from build123d import *

# Parameters (mm, degrees)
F0_R         = 6.35
F1_DEPTH     = 7.62
F2_W         = 7.62
F2_H         = 6.35
F3_DEPTH     = 25.4
F5_DEPTH     = 25.4
F7_DEPTH     = 63.5
F9_DEPTH     = 20.32
F11_DEPTH    = 25.4
F12_R        = 5.08
F13_R        = 0.508
F14_T1_DEPTH = 46.4482991577
F16_DEPTH    = 5.08
F18_DEPTH    = 1.27
F19_T4_DEPTH = 19.0509661188
F20_R        = 0.254


# Not quite as in the source:
# - a fillet or chamfer that OpenCascade refuses, or shapes differently, is made with other operations: its cross-section is extruded or revolved along the edge and cut away or added


with BuildPart() as f1:
    # F0 (on Front) → F1 (new body)
    with BuildSketch(Plane.XZ):
        with BuildLine():
            Line((15.24, 3.81), (9.4185720786, 3.81))
            ThreePointArc((9.4185720786, 3.81), (-10.16, 0), (9.4185720786, -3.81))
            Line((9.4185720786, -3.81), (15.24, -3.81))
            Line((15.24, -3.81), (15.24, 0))
            Line((15.24, 0), (15.24, 3.81))
        make_face()
        Circle(F0_R, mode=Mode.SUBTRACT)
    extrude(amount=F1_DEPTH)

    # F2 (on face) → F3 (join)
    with BuildSketch(Plane.YZ.offset(15.24)):
        Polygon((-7.62, 10.16), (-7.62, 3.81), (-15.24, 3.81), (-15.24, -10.16), (15.24, -10.16), (15.24, 3.81), (15.24, 10.16), align=None)
        with Locations((-11.43, 6.985)):
            Rectangle(F2_W, F2_H)
    extrude(amount=F3_DEPTH)

    # F4 (on face) → F5 (cut)
    with BuildSketch(Plane.XY.offset(10.16)):
        Polygon((31.65983, 15.24), (40.64, 15.24), (40.64, 6.25983), (47.585287597, 13.2393133827), (38.6222154898, 22.2023854898), align=None)
        Polygon((40.64, 6.25983), (40.64, 15.24), (31.65983, 15.24), align=None)
        with BuildLine():
            Line((40.64, 6.25983), (31.65983, 15.24))
            Line((31.65983, 15.24), (22.6795738789, 6.2597438789))
            ThreePointArc((22.6795738789, 6.2597438789), (22.6795738789, -2.7204261211), (31.6597438789, -2.7204261211))
            Line((31.6597438789, -2.7204261211), (40.64, 6.25983))
        make_face()
    extrude(amount=-F5_DEPTH, mode=Mode.SUBTRACT)

    # F6 (on face) → F7 (cut, symmetric)
    with BuildSketch(Plane(origin=(8.209915, -8.209915, 0), x_dir=(0.7071067812, 0.7071067812, 0), z_dir=(0.7071067812, -0.7071067812, 0))):
        with BuildLine():
            ThreePointArc((26.8131878295, 0.635), (24.5681237992, -4.7850640303), (29.9881878295, -2.54))
            ThreePointArc((29.9881878295, -2.54), (29.0582518598, -0.2949359697), (26.8131878295, 0.635))
        make_face()
    extrude(amount=F7_DEPTH, both=True, mode=Mode.SUBTRACT)

    # F8 (on face) → F9 (join)
    with BuildSketch(Plane.XY.offset(10.16)):
        with BuildLine():
            Line((31.6597438789, -2.7204261211), (40.64, 6.25983))
            Line((40.64, 6.25983), (38.8439487758, 8.0558812242))
            Line((38.8439487758, 8.0558812242), (26.2716117366, -4.516455815))
            ThreePointArc((26.2716117366, -4.516455815), (29.177671493, -4.2544271062), (31.6597438789, -2.7204261211))
        make_face()
    extrude(amount=-F9_DEPTH)

    # F10 (on face) → F11 (cut)
    with BuildSketch(Plane(origin=(8.209915, -8.209915, 0), x_dir=(0.7071067812, 0.7071067812, 0), z_dir=(0.7071067812, -0.7071067812, 0))):
        with BuildLine():
            ThreePointArc((29.9881878295, -2.54), (29.0582518598, -0.2949359697), (26.8131878295, 0.635))
            ThreePointArc((26.8131878295, 0.635), (24.5681237992, -4.7850640303), (29.9881878295, -2.54))
        make_face()
    extrude(amount=F11_DEPTH, mode=Mode.SUBTRACT)

    # F12
    f12_edges = [f1.edges().sort_by_distance(p)[0] for p in [
        (40.64, -15.24, 0),
    ]]
    fillet(f12_edges, radius=F12_R)

    # F13
    f13_edges = [f1.edges().sort_by_distance(p)[0] for p in [
        (15.24, -3.81, 3.81),
        (15.24, -3.81, -3.81),
    ]]
    fillet(f13_edges, radius=F13_R)

    # F14: chamfer of 5.08 on 1 edges, made by hand

    # F14_s2 → F14_t1 (cut)
    with BuildSketch(Plane.XY.offset(-23.2241495789)):
        Polygon((15.24, 10.16), (20.32, 15.24), (15.24, 15.24), align=None)
    extrude(amount=F14_T1_DEPTH, mode=Mode.SUBTRACT)

    # F15 (on face) → F16 (join)
    with BuildSketch(Plane.XY.offset(10.16)):
        with BuildLine():
            Line((31.65983, 15.24), (28.3609535545, 15.24))
            Line((28.3609535545, 15.24), (21.4524150836, 8.3314615291))
            ThreePointArc((21.4524150836, 8.3314615291), (19.5659150525, -1.0873397162), (27.5316145271, -6.4557967708))
            Line((27.5316145271, -6.4557967708), (26.2716117366, -4.516455815))
            ThreePointArc((26.2716117366, -4.516455815), (21.1455728938, -0.2383537351), (22.6795738789, 6.2597438789))
            Line((22.6795738789, 6.2597438789), (31.65983, 15.24))
        make_face()
    extrude(amount=F16_DEPTH)

    # F17 (on face) → F18 (cut)
    with BuildSketch(Plane.XY.offset(10.16)):
        Polygon((21.4524150836, 8.3314615291), (28.3609535545, 15.24), (25.7178656757, 15.24), (19.4216053933, 9.3011604622), align=None)
    extrude(amount=-F18_DEPTH, mode=Mode.SUBTRACT)

    # F19: fillet of radius 5.08 on 1 edges, made by hand


with BuildPart() as f19_tool2:
    # F19_s3 → F19_t4 (new body)
    with BuildSketch(Plane(origin=(4.6185626358, -2.2053347891, 0), x_dir=(0, 0, 1), z_dir=(0.9024034915, -0.4308920265, 0))):
        with BuildLine():
            ThreePointArc((8.89, -20.1221187471), (9.2180951188, -18.3260675229), (10.16, -16.762014582))
            Line((10.16, -16.762014582), (10.0838, -16.6948124987))
            ThreePointArc((10.0838, -16.6948124987), (9.525, -16.660414582), (8.89, -16.660414582))
            Line((8.89, -16.660414582), (8.7884, -16.762014582))
            Line((8.7884, -16.762014582), (8.7884, -20.1221187471))
            Line((8.7884, -20.1221187471), (8.89, -20.1221187471))
        make_face()
    extrude(amount=F19_T4_DEPTH)

    split(bisect_by=Plane(origin=(6.5604767773, -6.5604767773, 0), x_dir=(0, 0, 1), z_dir=(-0.7071067812, 0.7071067812, 0)), keep=Keep.TOP)

    split(bisect_by=Plane(origin=(4.5012786836, -4.7721818404, 0), x_dir=(0, 0, 1), z_dir=(0.6861575418, -0.727452973, 0)), keep=Keep.TOP)


with BuildPart() as f1_1:
    add(f1.part)

    # F19_t1: union F19_tool2
    add(f19_tool2.part)

    # F20
    f20_edges = [f1_1.edges().sort_by_distance(p)[0] for p in [
        (23.880158, 13.506614, 8.89),
        (20.64155, 10.451852, 9.218095),
    ]]
    fillet(f20_edges, radius=F20_R)


solid = f1_1.part
Design review of the part built by this model. Coordinates are the model's own, in mm. A direction names the side the tool comes from. Round coordinates to 2 decimals unless told otherwise and drop trailing zeros. Write each loop counter-clockwise with the first axis right and the second up, starting at its lowest first coordinate (ties: lowest second). Pieces come first, ordered by that corner, then holes. Notation, with made-up numbers: (-7, -21.75) -> (40, -21.75) arc R28 cw to (40, 16.25) -> close; hole circle Ø11 at (13, 37.5). An arc over 180 degrees is marked (long way). One line per item, written item: value. Start each with the question number.
Q1. Add section B-B (y = 7.5). Give the boundary of the cut face in (x, z), then the cut area to 3 significant figures.
Q2. To check wall thickness, follow probe 1 along Z at (x, y) = (0, -2); probe 2 along Y at (x, z) = (-7, 1.25); probe 3 along Y at (x, z) = (23.5, -9). State the ranges of each line that lie inside material, in increasing order.
Q3. Insertion check: P1, Ø2.5, axis at x = 13, y = -3, coming from the +Z side; P2, Ø3, axis at y = 10, z = 11.5, coming from the +X side; P3, Ø3, axis at y = 9.5, z = -5.5, coming from the -X side. Each pin has a flat end and moves straight along its axis. Give the tip position at first contact, or say it passes through.
Q4. The part is to be moulded in two halves that separate along Y. For faces 1 (the face through (12, -4, -3.81)), 2 (the face through (32.65, 1.86, 0.14)), 3 (the face through (5, -7.62, 5)), 4 (the face through (22.8, 12.49, 9.66)), say which applies: pulls with the +Y half, pulls with the -Y half, needs draft (parallel to the pull), parting line crosses it, or undercut.
Q5. Add section A-A (x = 0). Give the boundary of the cut face in (y, z).
Q6. Tool access review of faces 5 (the face through (25, 13, 8.89)), 6 (the face through (19.513, -0.955, 12.664)), 7 (the face through (39.8, 7.1, 0.1)), 8 (the face through (27.11, 10.69, 2.36)): name each direction out of +Z, -Z, +X, -X, +Y, -Y from which nothing blocks a thin tool from reaching the whole face with its end or side.
Response:
1. outline: (15.24, -10.16) -> (23.92, -10.16) -> (23.92, 15.24) -> (20.72, 15.24) -> (20.72, 10.16) -> (15.24, 10.16) -> close; (38.29, -10.16) -> (39.4, -10.16) -> (39.4, 10.16) -> (38.29, 10.16) -> close
1. area: 215 mm^2
2. probe 1: z = -10.16 to -6.35, 6.35 to 10.16
2. probe 2: y = -7.62 to 0
2. probe 3: y = -15.24 to -3.41, 7.08 to 15.24
3. P1: stops at z = 3.81
3. P2: stops at x = 27.92
3. P3: stops at x = 15.24
4. face 1: needs draft
4. face 2: undercut
4. face 3: pulls with the -Y half
4. face 4: undercut
5. outline: (-7.62, -10.16) -> (0, -10.16) -> (0, -6.35) -> (-7.62, -6.35) -> close; (-7.62, 6.35) -> (0, 6.35) -> (0, 10.16) -> (-7.62, 10.16) -> close
6. face 5: +Z
6. face 6: +Z, -X
6. face 7: +Z, -Z, +X, +Y
6. face 8: +Z, -Z
